```python
from build123d import *

# Parameters (mm, degrees)
SKETCH_1_R          = 2.55
SKETCH_1_R_2        = 4
EXTRUDE_1_DEPTH     = 2.5
SKETCH_2_W          = 12
SKETCH_2_H          = 2.5
EXTRUDE_2_DEPTH     = 20
SKETCH_3_R          = 2.55
CUT_EXTRUDE_1_DEPTH = 20
FILLET_1_R          = 2.5
EXTRUDE_3_DEPTH     = 5
EXTRUDE_4_DEPTH     = 2
EXTRUDE_5_DEPTH     = 2
SKETCH_7_R          = 4
CUT_EXTRUDE_2_DEPTH = 45.161634934


with BuildPart() as part:
    # Эскиз1 → Бобышка-Вытянуть1 (new body)
    with BuildSketch(Plane(origin=(0, 0, 0), x_dir=(1, 0, 0), z_dir=(0, 1, 0))):
        with BuildLine():
            Line((2.5, 0), (9.5, 0))
            ThreePointArc((9.5, 0), (11.267766953, -0.732233047), (12, -2.5))
            Line((12, -2.5), (12, -32))
            ThreePointArc((12, -32), (10.389087297, -35.889087297), (6.5, -37.5))
            Line((6.5, -37.5), (5.5, -37.5))
            ThreePointArc((5.5, -37.5), (1.610912703, -35.889087297), (0, -32))
            Line((0, -32), (0, -2.5))
            ThreePointArc((0, -2.5), (0.732233047, -0.732233047), (2.5, 0))
        make_face()
        with Locations(Location((6, -10, 0), (0, 0, 270))):
            Circle(SKETCH_1_R, mode=Mode.SUBTRACT)
        with Locations(Location((6, -31, 0), (0, 0, 270))):
            Circle(SKETCH_1_R_2, mode=Mode.SUBTRACT)
    extrude(amount=EXTRUDE_1_DEPTH)

    # Эскиз2 → Бобышка-Вытянуть2 (add)
    with BuildSketch(Plane(origin=(0, 2.5, 0), x_dir=(1, 0, 0), z_dir=(0, 1, 0))):
        with Locations((6, -21.25)):
            Rectangle(SKETCH_2_W, SKETCH_2_H)
    extrude(amount=EXTRUDE_2_DEPTH)

    # Эскиз3 → Вырез-Вытянуть1 (cut)
    with BuildSketch(Plane.XY.offset(22.5)):
        with Locations((6, 12.5)):
            Circle(SKETCH_3_R)
    extrude(amount=-CUT_EXTRUDE_1_DEPTH, mode=Mode.SUBTRACT)

    # Скругление1
    fillet_1_edges = [part.edges().sort_by_distance(p)[0] for p in [
        (0, 22.5, 21.25),
        (12, 22.5, 21.25),
    ]]
    fillet(fillet_1_edges, radius=FILLET_1_R)

    # Эскиз4 → Бобышка-Вытянуть3 (add)
    with BuildSketch(Plane(origin=(0, 2.5, 0), x_dir=(1, 0, 0), z_dir=(0, 1, 0))):
        with BuildLine():
            Line((12, -22.5), (0, -22.5))
            Line((0, -22.5), (0, -32))
            ThreePointArc((0, -32), (1.610912703, -35.889087297), (5.5, -37.5))
            Line((5.5, -37.5), (6.5, -37.5))
            ThreePointArc((6.5, -37.5), (10.389087297, -35.889087297), (12, -32))
            Line((12, -32), (12, -22.5))
        make_face()
    extrude(amount=EXTRUDE_3_DEPTH)

    # Эскиз5 → Бобышка-Вытянуть4 (add)
    with BuildSketch(Plane(origin=(12, 0, 0), x_dir=(0, 0, -1), z_dir=(1, 0, 0))):
        Polygon((-32, 7.5), (-22.5, 7.5), (-22.5, 20), align=None)
    extrude(amount=-EXTRUDE_4_DEPTH)

    # Эскиз6 → Бобышка-Вытянуть5 (add)
    with BuildSketch(Plane.ZY):
        Polygon((32, 7.5), (22.5, 20), (22.5, 7.5), align=None)
    extrude(amount=-EXTRUDE_5_DEPTH)

    # Эскиз7 → Вырез-Вытянуть2 (cut, through all)
    with BuildSketch(Plane.XZ.offset(-2.5)):
        with Locations(Location((6, 31, 0), (0, 0, 180))):
            Circle(SKETCH_7_R)
    extrude(amount=-CUT_EXTRUDE_2_DEPTH, mode=Mode.SUBTRACT)


solid = part.part
```
Check sheet for the modelled part. Datum: model origin and axes. Units: mm. A direction names the side the tool comes from. Coordinates: 2 decimals unless noted, no trailing zeros. Loops run counter-clockwise (first coordinate to the right, second up) from the corner with the lowest first, then second, coordinate; pieces in that order, holes last.
1) Gauge pin test, flat ends, axial feed: pin 1 (6 mm diameter, centred on x = 6, y = 12.5, fed in from +Z); pin 2 (6 mm diameter, centred on x = 6.5, y = 15, fed in from -Z); pin 3 (5 mm diameter, centred on x = 4.5, z = 33, fed in from +Y). Record the tip position at first contact, or that the pin passes through.
2) Access from +Z, -Z, +X, -X, +Y, -Y to the whole of each face (thin tool, end or side, straight path). Record for faces 4 (the face through (4.6, 10.1, 20)), 5 (the face through (2, 11, 25)), 6 (the face through (7.18, 10.24, 21.27)).
3) Release check for a two-part mould opening along Z. For faces 1 (the face through (6.77, 1.23, 12.43)), 2 (the face through (6, 7.5, 36)), 3 (the face through (0.99, 13.66, 27.32)) record: released by +Z, released by -Z, zero draft, split by the parting line, or undercut.
4) Material ranges on probe 1 along X at (y, z) = (3.9, 31); probe 2 along Y at (x, z) = (6, 21.75); probe 3 along Y at (x, z) = (8.75, 2), recorded low to high.
5) Sectioned sample at B-B (y = 4.5). Record the boundary of the cut face in (x, z), and give its area (3 significant figures).
6) Sectioned sample at A-A (x = 6). Record the boundary of the cut face in (y, z).
7) Sectioned sample at C-C (z = 10.5). Record the boundary of the cut face in (x, y).
8) Sectioned sample at D-D (y = 12.5). Record the boundary of the cut face in (x, z), and give its area (4 significant figures).
Check sheet entries:
1. pin 1: stops at z = 22.5
1. pin 2: stops at z = 20
1. pin 3: stops at y = 7.5
2. face 4: -Z, +X, -X, +Y
2. face 5: +Z, +Y
2. face 6: +Z, -Z
3. face 1: undercut
3. face 2: zero draft
3. face 3: released by +Z
4. probe 1: x = 0 to 2, 10 to 12
4. probe 2: y = 0 to 9.95, 15.05 to 22.5
4. probe 3: y = 0 to 2.5
5. outline: (0, 20) - (12, 20) - (12, 32) arc R5.5 ccw to (6.5, 37.5) - (5.5, 37.5) arc R5.5 ccw to (0, 32) - close; hole circle Ø8 at (6, 31)
5. area: 147 mm2
6. outline: (0, 0) - (2.5, 0) - (2.5, 7.45) - (0, 7.45) - close; (0, 12.55) - (2.5, 12.55) - (2.5, 20) - (9.95, 20) - (9.95, 22.5) - (7.5, 22.5) - (7.5, 27) - (0, 27) - close; (0, 35) - (7.5, 35) - (7.5, 37.5) - (0, 37.5) - close; (15.05, 20) - (22.5, 20) - (22.5, 22.5) - (15.05, 22.5) - close
7. outline: (0, 0) - (3.5, 0) - (3.5, 2.5) - (0, 2.5) - close; (8.5, 0) - (12, 0) - (12, 2.5) - (8.5, 2.5) - close
8. outline: (0, 20) - (3.45, 20) - (3.45, 22.5) - (2, 22.5) - (2, 28.2) - (0, 28.2) - close; (8.55, 20) - (12, 20) - (12, 28.2) - (10, 28.2) - (10, 22.5) - (8.55, 22.5) - close
8. area: 40.05 mm2
